For this review, use the dimensioned drawing (mm, ordinates from the lowest corner) and the shaded views. A direction names the side the tool comes from. Give positions to 0.01 mm unless a question says otherwise; leave off trailing zeros. Loops run counter-clockwise (first coordinate to the right, second up) from the corner with the lowest first, then second, coordinate; pieces in that order, holes last. Notation, with made-up numbers: (47.25, 7) -> (85.25, 7) arc R23 ccw to (85.25, 46) -> close; hole circle Ø3 at (54, 40.25). An arc over 180 degrees is marked (long way). Write each question's results on one line, items separated by ' | '. Start each with the question number.
Q1. Machinability: for the marked faces 4 and 5, which of the approach directions +Z, -Z, +X, -X, +Y, -Y give a long, thin tool a straight path to every point of the face, cutting with its end or side? Answer none if there is none.
Q2. Wall thickness on L1, parallel to X at y = 2.35, z = 8.25; L2, parallel to Z at x = 9.25, y = 0.2: over which ranges is each line inside the solid? List them lowest first. Write a range as [from, to].
Q3. Insertion check: pin 1 Ø1.5 at (x, y) = (6.5, 1.5) entering from +Z; pin 2 Ø1.5 at (x, y) = (8, 2.5) entering from -Z. Each pin has a flat end and moves straight along its axis. Give the tip position at first contact, or say it passes through.
Q4. We need section A-A (z = 4.25). Write out the cut boundary in (x, y).
Q5. We need section B-B (y = 1.95). Write out the cut boundary in (x, z), plus the area to 3 significant figures.
Q6. Mouldability with a two-part tool opening along X and no side actions: class the marked faces 1, 2 and 3 as released by +X, released by -X, zero draft, split by the parting line, or undercut.
Q7. We need section C-C (x = 5.25). Write out the cut boundary in (y, z), plus the area to 3 significant figures.
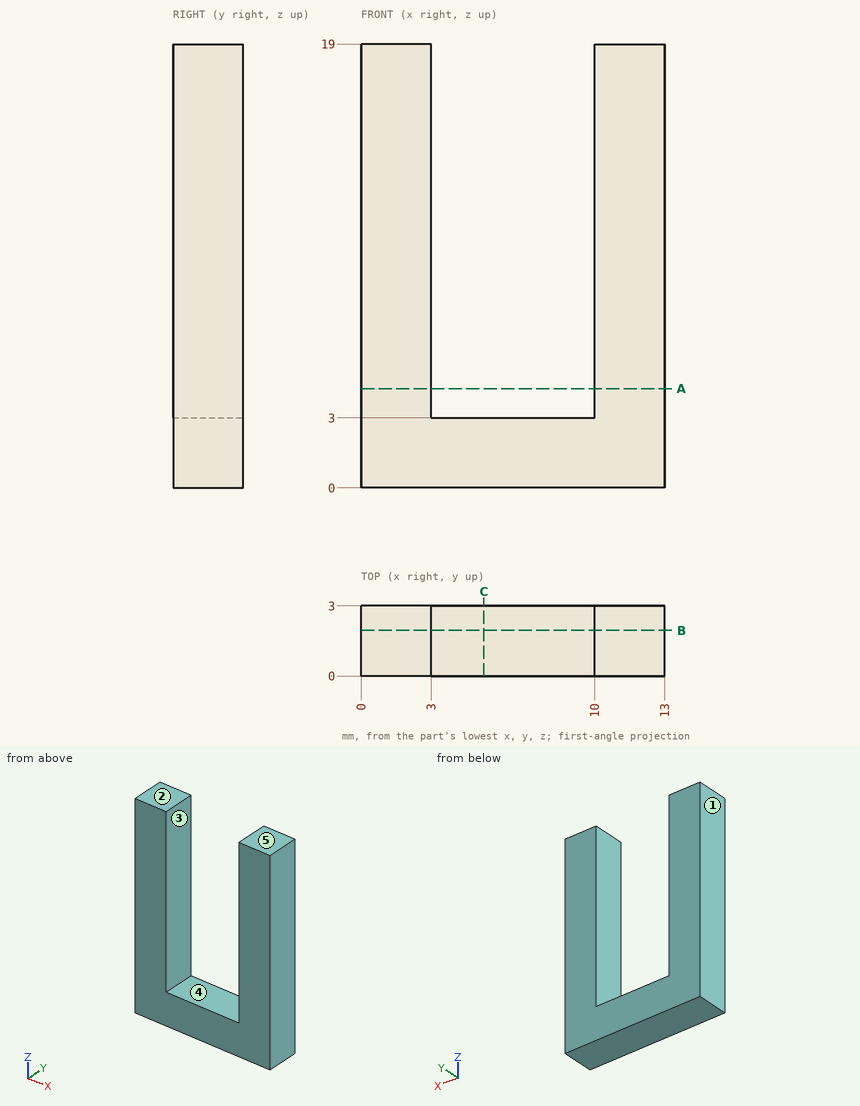
Output:
1) face 4: +Z, +Y, -Y | face 5: +Z, +X, -X, +Y, -Y
2) L1: [0, 3], [10, 13] | L2: [0, 3]
3) pin 1: z = 3 | pin 2: z = 0
4) outline: (0, 0) -> (3, 0) -> (3, 3) -> (0, 3) -> close; (10, 0) -> (13, 0) -> (13, 3) -> (10, 3) -> close
5) outline: (0, 0) -> (13, 0) -> (13, 19) -> (10, 19) -> (10, 3) -> (3, 3) -> (3, 19) -> (0, 19) -> close | area: 135 mm2
6) face 1: released by -X | face 2: zero draft | face 3: undercut
7) outline: (0, 0) -> (3, 0) -> (3, 3) -> (0, 3) -> close | area: 9.00 mm2
